CAD build for the part. Positions are in the model's coordinates, mm. A direction names the side the tool comes from. Round coordinates to 2 decimals unless told otherwise and drop trailing zeros. Write each loop counter-clockwise with the first axis right and the second up, starting at its lowest first coordinate (ties: lowest second). Pieces come first, ordered by that corner, then holes. Notation, with made-up numbers: (-36.75, 72.5) - (-8.75, 72.5) arc R21 cw to (-8.75, 109.5) - close; hole circle Ø4 at (61.5, -5.75). An arc over 180 degrees is marked (long way). Answer in a Markdown table with one row per item.
```python
from build123d import *

# Parameters (mm, degrees)
SCHIZZO1_W                   = 135
SCHIZZO1_H                   = 110
SCHIZZO1_R                   = 5
ESTRUSIONE_ESTRUSIONE1_DEPTH = 3


with BuildPart() as part:
    # Schizzo1 → Estrusione-Estrusione1 (new body)
    with BuildSketch(Plane.XY):
        Rectangle(SCHIZZO1_W, SCHIZZO1_H)
        with Locations((-52.5, 38.75)):
            Circle(SCHIZZO1_R, mode=Mode.SUBTRACT)
        with Locations((-52.5, -38.75)):
            Circle(SCHIZZO1_R, mode=Mode.SUBTRACT)
        with Locations((52.5, -38.75)):
            Circle(SCHIZZO1_R, mode=Mode.SUBTRACT)
        with Locations((52.5, 38.75)):
            Circle(SCHIZZO1_R, mode=Mode.SUBTRACT)
    extrude(amount=ESTRUSIONE_ESTRUSIONE1_DEPTH)

    # Schizzo3 → Rivoluzione1 (revolve)
    with BuildSketch(Plane(origin=(0, 0, 0), x_dir=(1, 0, 0), z_dir=(0, 1, 0))):
        Polygon((47.25, -4), (49.75, -6.5), (49.75, -14.66), (47.25, -17.16), (46.5, -17.16), (46.5, -4), (36.5, -4), (36.5, -24.79), (0, -24.79), (0, -4), (0, -3), (47.25, -3), align=None)
    revolve(axis=Axis((0, 0, 4), (0, 0, -1)))


solid = part.part
```
Q1. Pull direction X, two halves, no side cores. Call faces 4 (the flat face through (-1, 1, 0)), 5 (the conical face through (45.18, -14.23, 17.04)), 6 (the flat face through (-28, 24, 4)): released by +X, released by -X, zero draft, split by the parting line, or undercut.
Computed:
| item | result |
|---|---|
| face 4 | zero draft |
| face 5 | split by the parting line |
| face 6 | undercut |
Q2. Drill centre lines: line 1 (Y direction, x = 52.5, z = 0.9); line 2 (X direction, y = -23, z = 16.25); line 3 (Y direction, x = 0, z = 9.75). Where is each one in solid material? Low to high.
Computed:
| item | result |
|---|---|
| line 1 | y = -55 to -43.75, -33.75 to 33.75, 43.75 to 55 |
| line 2 | x = -42.31 to -40.41, -28.34 to 28.34, 40.41 to 42.31 |
| line 3 | y = -49.75 to -46.5, -36.5 to 36.5, 46.5 to 49.75 |
Q3. 3-axis set-ups, long thin cutter, end or side, ignore diameter. For faces 1 (the flat face through (-1, 55, 1)), 2 (the cylindrical face through (-7.912, 35.632, 14.541)), 3 (the flat face through (-46, 13, 3)): which of +Z, -Z, +X, -X, +Y, -Y reach the whole face in a straight line?
Computed:
| item | result |
|---|---|
| face 1 | +Z, -Z, +X, -X, +Y |
| face 2 | +Z |
| face 3 | none |
Q4. Saw through at A-A on x = -52.5. List the corners of the cut face in (y, z), then the cut area to 3 significant figures.
Computed:
| item | result |
|---|---|
| outline | (-55, 0) - (-43.75, 0) - (-43.75, 3) - (-55, 3) - close; (-33.75, 0) - (33.75, 0) - (33.75, 3) - (-33.75, 3) - close; (43.75, 0) - (55, 0) - (55, 3) - (43.75, 3) - close |
| area | 270 mm2 |
Q5. Flat gauge pins, fed straight in: pin 1 (4 mm diameter, centred on y = 1, z = 8.5, fed in from +X); pin 2 (10 mm diameter, centred on x = -3, z = 17.5, fed in from +Y); pin 3 (4 mm diameter, centred on x = 47.5, z = 12, fed in from +Y). Where does each tip first touch, or does it go through?
Computed:
| item | result |
|---|---|
| pin 1 | stops at x = 49.75 |
| pin 2 | stops at y = 49.75 |
| pin 3 | stops at y = 20.12 |
Q6. Saw through at C-C on y = 38.75. Count the separate pieces of the cut face and the enclosed holes in it, then the cut area to 3 significant figures.
Computed:
| item | result |
|---|---|
| separate pieces | 3 |
| enclosed holes | 0 |
| area | 523 mm2 |
Q7. Saw through at B-B on z = 10.75. List the corners of the cut face in (x, y), then the cut area to 3 significant figures.
Computed:
| item | result |
|---|---|
| outline | circle Ø99.5 at (0, 0); circle Ø73 at (0, 0); hole circle Ø93 at (0, 0) |
| area | 5,170 mm2 |
